Check sheet for the modelled part. Datum: model origin and axes. Units: mm. A direction names the side the tool comes from. Round coordinates to 2 decimals unless told otherwise and drop trailing zeros. Write each loop counter-clockwise with the first axis right and the second up, starting at its lowest first coordinate (ties: lowest second). Pieces come first, ordered by that corner, then holes.
Autodesk Inventor part; units mm, degrees
ref_plane "YZ Plane" through (0, 0, 0) normal (1, 0, 0) x (0, 1, 0)
ref_plane "XZ Plane" through (0, 0, 0) normal (0, 1, 0) x (-1, 0, 0)
ref_plane "XY Plane" through (0, 0, 0) normal (0, 0, 1) x (1, 0, 0)
sketch "Sketch1" plane through (0, 0, 0) normal (1, 0, 0) x (0, 1, 0)
  circle A0 centre (0, 0) radius 7
  dimension "d0" = 14
extrude "Extrusion1" add sketch "Sketch1" along normal blind 17
sketch "Sketch2" plane through (17, 0, 0) normal (1, 0, 0) x (0, 0, -1)
  line L0 (-10.15, -10.15) -> (10.15, -10.15)
  line L1 (10.15, -10.15) -> (10.15, 10.15)
  line L2 (10.15, 10.15) -> (-10.15, 10.15)
  line L3 (-10.15, 10.15) -> (-10.15, -10.15)
  line L4 (-10.15, -10.15) -> (10.15, 10.15) construction
  line L5 (10.15, -10.15) -> (-10.15, 10.15) construction
  point P0 (0, 0)
  dimension "d3" = 20.3
  dimension "d4" = 20.3
extrude "Extrusion2" add sketch "Sketch2" along normal blind 6
sketch "Sketch3" plane through (23, 0, 0) normal (1, 0, 0) x (0, 0, -1)
  arc A0 (-10.98, 2.1499) -> (-10.98, -2.1501) centre (-10.98, -0.0001) ccw
  arc A1 (11.02, -2.1497) -> (10.98, 2.1499) centre (11.02, 0.0003) ccw
  line L0 (10.15, -10.15) -> (10.15, 10.15)
  line L1 (-10.15, 10.15) -> (-10.15, -10.15)
  line L2 (-10.98, 2.1499) -> (-10.15, 2.1499)
  line L3 (-10.98, -2.1501) -> (-10.15, -2.1501)
  line L4 (10.98, 2.1499) -> (10.15, 2.1499)
  line L5 (11.02, -2.1497) -> (10.15, -2.1497)
  line L6 (-10.15, 2.1499) -> (-10.15, -2.1501)
  line L7 (10.15, 2.1499) -> (10.15, -2.1497)
  point P0 (0, 0)
  dimension "d7" = 4.3
  dimension "d8" = 4.3
  dimension "d13" = 22
extrude "Extrusion3" add sketch "Sketch3" against normal up to surface (6 mm away)
properties part number "camera_Fatshark_600TVL"
1. Sectioned sample at D-D, the plane x = 14.5. Enter the section's corners in (y, z), plus the area to 3 significant figures.
2. Sectioned sample at B-B, the plane z = 0. Enter the section's corners in (x, y), plus the area to 3 significant figures.
3. Go/stop test with flat-tipped pins: pin 1 (3 mm diameter, centred on x = 20, y = -7, fed in from +Z); pin 2 (1.5 mm diameter, centred on x = 14.5, y = 5, fed in from +Z); pin 3 (3 mm diameter, centred on x = 20, y = -5.5, fed in from -Z). Record where each tip stops, or that it passes through.
4. Sectioned sample at C-C, the plane x = 19.5. Enter the section's corners in (y, z), plus the area to 3 significant figures.
5. Set-up check for faces 1 (the flat face through (20, 6, -10.15)), 2 (the flat face through (20, -6, -10.15)), 3 (the flat face through (20, -2.15, 10.6)): record each of +Z, -Z, +X, -X, +Y, -Y from which the full face is reachable in a straight line by a thin tool's end or side.
6. Sectioned sample at A-A, the plane y = 0. Enter the section's corners in (x, z), plus the area to 3 significant figures.
7. Scan lines: line 1 along X through (y, z) = (-8.25, 9.5); line 2 along Z through (x, y) = (18.75, 7); line 3 along Z through (x, y) = (8, 5.75). Record each from-to range of solid material in increasing order.
Computed values:
1. outline: circle Ø14 at (0, 0)
1. area: 154 mm2
2. outline: (0, -7) - (17, -7) - (17, -10.15) - (23, -10.15) - (23, 10.15) - (17, 10.15) - (17, 7) - (0, 7) - close
2. area: 360 mm2
3. pin 1: stops at z = 10.15
3. pin 2: stops at z = 5.56
3. pin 3: stops at z = -10.15
4. outline: (-10.15, -10.15) - (-2.15, -10.15) - (-2.15, -11.02) arc R2.15 ccw (long way) to (2.15, -10.98) - (2.15, -10.15) - (10.15, -10.15) - (10.15, 10.15) - (2.15, 10.15) - (2.15, 10.98) arc R2.15 ccw to (-2.15, 10.98) - (-2.15, 10.15) - (-10.15, 10.15) - close
4. area: 434 mm2
5. face 1: -Z, +X, -X, +Y
5. face 2: -Z, +X, -X, -Y
5. face 3: +Z, +X, -X, -Y
6. outline: (0, -7) - (17, -7) - (17, -13.17) - (23, -13.17) - (23, 13.13) - (17, 13.13) - (17, 7) - (0, 7) - close
6. area: 396 mm2
7. line 1: x = 17 to 23
7. line 2: z = -10.15 to 10.15
7. line 3: z = -3.99 to 3.99
